Read the model definition and answer for the solid it produces. Units are mm, in the model's axes. A direction names the side the tool comes from. Give positions to 0.01 mm unless a question says otherwise; leave off trailing zeros. Order: outer loops, then holes, each group sorted by start corner. A loop starts at its lowest first (then second) coordinate and runs counter-clockwise, first axis right, second up. Notation, with made-up numbers: (-28, -10) - (-17, -10) arc R27 ccw to (-17, 29) - close; hole circle Ø11 at (87, 18). An arc over 180 degrees is marked (long way). Use a Markdown table: item, result. Add a question column.
1. A cutting plane is placed at B-B on z = 5. Determine the outline of the cut face in (x, y).
2. Consider L1, parallel to X at y = 0.6, z = 4.25; L2, parallel to X at y = 1.55, z = 5; L3, parallel to X at y = 2.85, z = 2.75. Determine where each line is inside the solid, lowest interval first.
3. A cutting plane is placed at A-A on x = 5. Determine the outline of the cut face in (y, z), and give its area (3 significant figures).
4. A cutting plane is placed at D-D on z = 1.5. Determine the outline of the cut face in (x, y).
5. For a pull along Z with two mould halves and no side action, classify faces 3 (the flat face through (15, 4, 0)), 4 (the cylindrical face through (3.58, 2.54, 5.74)), 5 (the flat face through (15, 5, 5)) as released by +Z, released by -Z, zero draft, split by the parting line, or undercut.
6. A flat-ended cylindrical pin translates along its axis: P1, Ø1, axis at x = 21, z = 8, coming from the -Y side. Find the tip coordinate at first contact, or state that the pin passes through.
7. A cutting plane is placed at C-C on y = 4.6. Determine the outline of the cut face in (x, z).
8. Which of the six approach directions +Z, -Z, +X, -X, +Y, -Y give full straight-line access (tool end or side, diameter ignored) to faces 1 (the cylindrical face through (20.347, 0.317, 5.07)), 2 (the flat face through (27, 0, 5))?
```python
from build123d import *

# Parameters (mm, degrees)
AUFSATZ_LINEAR_AUSTRAGEN1_DEPTH = 10
SKIZZE4_R                       = 1.6
SCHNITT_LINEAR_AUSTRAGEN1_DEPTH = 10
FASE1_SIZE                      = 3
VERRUNDUNG1_R                   = 3


with BuildPart() as part:
    # Skizze3 → Aufsatz-Linear austragen1 (new body)
    with BuildSketch(Plane.XY):
        with BuildLine():
            Line((0, 0), (0, 5))
            Line((0, 5), (30, 5))
            Line((30, 5), (30, 0))
            Line((30, 0), (20, 0))
            ThreePointArc((20, 0), (15, 3.289673338), (10, 0))
            Line((10, 0), (0, 0))
        make_face()
    extrude(amount=AUFSATZ_LINEAR_AUSTRAGEN1_DEPTH)

    # Skizze4 → Schnitt-Linear austragen1 (cut)
    with BuildSketch(Plane(origin=(0, 5, 0), x_dir=(1, 0, 0), z_dir=(0, 1, 0))):
        with Locations(Location((5, -5, 0), (0, 0, 270))):
            Circle(SKIZZE4_R)
        with Locations(Location((25, -5, 0), (0, 0, 270))):
            Circle(SKIZZE4_R)
    extrude(amount=-SCHNITT_LINEAR_AUSTRAGEN1_DEPTH, mode=Mode.SUBTRACT)

    # Fase1
    fase1_edges = [part.edges().sort_by_distance(p)[0] for p in [
        (0, 5, 5),
        (30, 5, 5),
    ]]
    chamfer(fase1_edges, length=FASE1_SIZE)

    # Verrundung1
    verrundung1_edges = [part.edges().sort_by_distance(p)[0] for p in [
        (20, 0, 5),
        (10, 0, 5),
    ]]
    fillet(verrundung1_edges, radius=VERRUNDUNG1_R)


solid = part.part
```
Output values:
| question | item | result |
|---|---|---|
| 1 | outline | (0, 0) - (3.4, 0) - (3.4, 5) - (3, 5) - (0, 2) - close; (6.6, 0) - (8.31, 0) arc R3 ccw to (10.69, 1.17) arc R5.44 cw to (19.31, 1.17) arc R3 ccw to (21.69, 0) - (23.4, 0) - (23.4, 5) - (6.6, 5) - close; (26.6, 0) - (30, 0) - (30, 2) - (27, 5) - (26.6, 5) - close |
| 2 | L1 | 0 to 3.59, 6.41 to 10.11, 19.89 to 23.59, 26.41 to 30 |
| 2 | L2 | 0 to 3.4, 6.6 to 11.01, 18.99 to 23.4, 26.6 to 30 |
| 2 | L3 | 0.85 to 12.86, 17.14 to 29.15 |
| 3 | outline | (0, 0) - (5, 0) - (5, 3.4) - (0, 3.4) - close; (0, 6.6) - (5, 6.6) - (5, 10) - (0, 10) - close |
| 3 | area | 34.0 mm² |
| 4 | outline | (0, 0) - (8.31, 0) arc R3 ccw to (10.69, 1.17) arc R5.44 cw to (19.31, 1.17) arc R3 ccw to (21.69, 0) - (30, 0) - (30, 2) - (27, 5) - (3, 5) - (0, 2) - close |
| 5 | face 3 | released by -Z |
| 5 | face 4 | undercut |
| 5 | face 5 | zero draft |
| 6 | P1 | y = 0.01 |
| 7 | outline | (2.6, 0) - (27.4, 0) - (27.4, 10) - (2.6, 10) - close; hole circle Ø3.2 at (5, 5); hole circle Ø3.2 at (25, 5) |
| 8 | face 1 | +Z, -Z, -Y |
| 8 | face 2 | +Z, -Z, +X, -X, -Y |
